Check sheet for the modelled part. Datum: model origin and axes. Units: mm. A direction names the side the tool comes from. Round coordinates to 2 decimals unless told otherwise and drop trailing zeros. Order: outer loops, then holes, each group sorted by start corner. A loop starts at its lowest first (then second) coordinate and runs counter-clockwise, first axis right, second up. Notation, with made-up numbers: (71.5, 37) -> (123.5, 37) arc R15 cw to (123.5, 48) -> close; hole circle Ø8 at (88, 51). An arc over 180 degrees is marked (long way). Use CSV: the item, a comma, the result in double quotes.
```python
from build123d import *

# Parameters (mm, degrees)
SKETCH2_R           = 14
BOSS_EXTRUDE1_DEPTH = 4
SKETCH1_W           = 8
SKETCH1_H           = 22.649954628
SKETCH1_W_2         = 6
SKETCH1_H_2         = 18.4
BOSS_EXTRUDE2_DEPTH = 18
SKETCH3_W           = 8
SKETCH3_H           = 22.649954628
BOSS_EXTRUDE3_DEPTH = 2
SKETCH4_W           = 6
SKETCH4_H           = 18.4
CUT_EXTRUDE1_DEPTH  = 29.142494559
SKETCH5_W           = 5
SKETCH5_H           = 18.4
CUT_EXTRUDE2_DEPTH  = 33.57299495
SKETCH11_W          = 8
SKETCH11_H          = 18.310644234
BOSS_EXTRUDE5_DEPTH = 5.5
BOSS_EXTRUDE4_DEPTH = 25.5
CUT_EXTRUDE4_START  = 5.5
SKETCH9_W           = 3.5
SKETCH9_H           = 7
CUT_EXTRUDE4_DEPTH  = 6
SKETCH7_R           = 0.75
CUT_EXTRUDE5_DEPTH  = 41.03022536
FILLET3_R           = 1
FILLET4_R           = 2
FILLET5_R           = 2
SKETCH14_W          = 1.5
SKETCH14_H          = 2
FILLET6_R           = 2


# Some blends are built 0.0001 mm under size
with BuildPart() as part:
    # Sketch2 → Boss-Extrude1 (new body)
    with BuildSketch(Plane.XY):
        Circle(SKETCH2_R)
    extrude(amount=BOSS_EXTRUDE1_DEPTH)

    # Sketch1 → Boss-Extrude2 (add)
    with BuildSketch(Plane.XY.offset(4)):
        Rectangle(SKETCH1_W, SKETCH1_H)
        Rectangle(SKETCH1_W_2, SKETCH1_H_2, mode=Mode.SUBTRACT)
    extrude(amount=BOSS_EXTRUDE2_DEPTH)

    # Sketch3 → Boss-Extrude3 (add)
    with BuildSketch(Plane.XY.offset(22)):
        Rectangle(SKETCH3_W, SKETCH3_H)
    extrude(amount=BOSS_EXTRUDE3_DEPTH)

    # Sketch4 → Cut-Extrude1 (cut, through all)
    with BuildSketch(Plane.XY.offset(4)):
        Rectangle(SKETCH4_W, SKETCH4_H)
    extrude(amount=-CUT_EXTRUDE1_DEPTH, mode=Mode.SUBTRACT)

    # Sketch5 → Cut-Extrude2 (cut, through all)
    with BuildSketch(Plane.ZY.offset(-3)):
        with Locations((19.5, 0)):
            Rectangle(SKETCH5_W, SKETCH5_H)
    extrude(amount=CUT_EXTRUDE2_DEPTH, mode=Mode.SUBTRACT)

    # Sketch11 → Boss-Extrude5 (add)
    with BuildSketch(Plane.XY.offset(24)):
        Rectangle(SKETCH11_W, SKETCH11_H)
    extrude(amount=BOSS_EXTRUDE5_DEPTH)

    # Sketch8 → Boss-Extrude4 (add)
    with BuildSketch(Plane.XY.offset(4)):
        with BuildLine():
            Line((4, 11.324977314), (4, -11.324977314))
            Line((4, -11.324977314), (8.23072833, -11.324977314))
            ThreePointArc((8.23072833, -11.324977314), (12.474578081, -6.354911619), (14, 0))
            ThreePointArc((14, 0), (12.474578081, 6.354911619), (8.23072833, 11.324977314))
            Line((8.23072833, 11.324977314), (4, 11.324977314))
        make_face()
    extrude(amount=BOSS_EXTRUDE4_DEPTH)

    # Sketch9 → Cut-Extrude4 (cut)
    with BuildSketch(Plane.XY.offset(24).offset(CUT_EXTRUDE4_START)):
        with Locations((5.75, 0)):
            Rectangle(SKETCH9_W, SKETCH9_H)
    extrude(amount=-CUT_EXTRUDE4_DEPTH, mode=Mode.SUBTRACT)

    # Sketch7 → Cut-Extrude5 (cut, through all)
    with BuildSketch(Plane(origin=(0, -9.155322117, 0), x_dir=(1, 0, 0), z_dir=(0, 1, 0))):
        with Locations((0, -26.75)):
            Circle(SKETCH7_R)
    extrude(amount=CUT_EXTRUDE5_DEPTH, mode=Mode.SUBTRACT)

    # Fillet3
    fillet3_edges = [part.edges().sort_by_distance(p)[0] for p in [
        (-4, -9.2, 19.5),
        (-4, 0, 17),
        (-4, 9.2, 19.5),
    ]]
    fillet(fillet3_edges, radius=FILLET3_R - 0.0001)  # a hair under: the kernel refuses the full size

    # Fillet4
    # the kernel refuses this fillet: 2 mm, written as the material it adds along each edge
    with BuildSketch(Plane(origin=(13.23072833, -11.324977314, 4), x_dir=(0, -1, 0), z_dir=(-1, 0, 0))) as fillet4_piece_1_section:
        with BuildLine():
            CenterArc((FILLET4_R, FILLET4_R), FILLET4_R, 180, 90)
            Line((0, FILLET4_R), (0, 0))
            Line((0, 0), (FILLET4_R, 0))
        make_face()
    fillet4_piece_1 = extrude(amount=17.23072833, mode=Mode.PRIVATE)
    fillet4_piece_1 = fillet4_piece_1 & Plane(origin=(0, 0, 4.46853923), x_dir=(1, 0, 0), z_dir=(0, 0, -1)) * Cylinder(14, 43, mode=Mode.PRIVATE)
    add(fillet4_piece_1)
    with BuildSketch(Plane(origin=(-4, 11.324977314, 4), x_dir=(0, 0, 1), z_dir=(0, -1, 0))) as fillet4_piece_2:
        with BuildLine():
            CenterArc((FILLET4_R, FILLET4_R), FILLET4_R, 180, 90)
            Line((0, FILLET4_R), (0, 0))
            Line((0, 0), (FILLET4_R, 0))
        make_face()
    extrude(amount=22.649954628)
    with BuildSketch(Plane(origin=(-4, 11.324977314, 4), x_dir=(0, 1, 0), z_dir=(1, 0, 0))) as fillet4_piece_3_section:
        with BuildLine():
            CenterArc((FILLET4_R, FILLET4_R), FILLET4_R, 180, 90)
            Line((0, FILLET4_R), (0, 0))
            Line((0, 0), (FILLET4_R, 0))
        make_face()
    fillet4_piece_3 = extrude(amount=17.23072833, mode=Mode.PRIVATE)
    fillet4_piece_3 = fillet4_piece_3 & Plane(origin=(0, 0, 4.468539385), x_dir=(1, 0, 0), z_dir=(0, 0, -1)) * Cylinder(14, 43, mode=Mode.PRIVATE)
    add(fillet4_piece_3)
    with BuildSketch(Plane(origin=(-4, 11.324977314, 4), x_dir=(0, 0, 1), z_dir=(0, -1, 0))) as fillet4_piece_4a_section:
        with BuildLine():
            CenterArc((FILLET4_R, FILLET4_R), FILLET4_R, 180, 90)
            Line((0, FILLET4_R), (0, 0))
            Line((0, 0), (FILLET4_R, 0))
        make_face()
    fillet4_piece_4a = extrude(amount=27.649954628, mode=Mode.PRIVATE)
    fillet4_piece_4a = split(fillet4_piece_4a, bisect_by=Plane(origin=(-4.418611248, -11.324977314, 4.472457753), z_dir=(0, -1, 0)), keep=Keep.TOP, mode=Mode.PRIVATE)
    fillet4_piece_4a = fillet4_piece_4a & Plane(origin=(0, 0, 4.472457753), x_dir=(1, 0, 0), z_dir=(0, 0, -1)) * Cylinder(14, 64, mode=Mode.PRIVATE)
    with BuildSketch(Plane(origin=(13.23072833, -11.324977314, 4), x_dir=(0, -1, 0), z_dir=(-1, 0, 0))) as fillet4_piece_4b_section:
        with BuildLine():
            CenterArc((FILLET4_R, FILLET4_R), FILLET4_R, 180, 90)
            Line((0, FILLET4_R), (0, 0))
            Line((0, 0), (FILLET4_R, 0))
        make_face()
    fillet4_piece_4b = extrude(amount=22.23072833, mode=Mode.PRIVATE)
    fillet4_piece_4b = split(fillet4_piece_4b, bisect_by=Plane(origin=(-4, -11.687205264, 4.504335867), z_dir=(-1, 0, 0)), keep=Keep.TOP, mode=Mode.PRIVATE)
    fillet4_piece_4b = fillet4_piece_4b & Plane(origin=(0, 0, 4.504335867), x_dir=(1, 0, 0), z_dir=(0, 0, -1)) * Cylinder(14, 53, mode=Mode.PRIVATE)
    fillet4_piece_4 = fillet4_piece_4a & fillet4_piece_4b
    add(fillet4_piece_4)
    with BuildSketch(Plane(origin=(-4, 16.324977314, 4), x_dir=(0, 0, 1), z_dir=(0, -1, 0))) as fillet4_piece_5a_section:
        with BuildLine():
            CenterArc((FILLET4_R, FILLET4_R), FILLET4_R, 180, 90)
            Line((0, FILLET4_R), (0, 0))
            Line((0, 0), (FILLET4_R, 0))
        make_face()
    fillet4_piece_5a = extrude(amount=27.649954628, mode=Mode.PRIVATE)
    fillet4_piece_5a = split(fillet4_piece_5a, bisect_by=Plane(origin=(-4.418615633, 11.324977314, 4.472459709), z_dir=(0, 1, 0)), keep=Keep.TOP, mode=Mode.PRIVATE)
    fillet4_piece_5a = fillet4_piece_5a & Plane(origin=(0, 0, 4.472459709), x_dir=(1, 0, 0), z_dir=(0, 0, -1)) * Cylinder(14, 64, mode=Mode.PRIVATE)
    with BuildSketch(Plane(origin=(-9, 11.324977314, 4), x_dir=(0, 1, 0), z_dir=(1, 0, 0))) as fillet4_piece_5b_section:
        with BuildLine():
            CenterArc((FILLET4_R, FILLET4_R), FILLET4_R, 180, 90)
            Line((0, FILLET4_R), (0, 0))
            Line((0, 0), (FILLET4_R, 0))
        make_face()
    fillet4_piece_5b = extrude(amount=22.23072833, mode=Mode.PRIVATE)
    fillet4_piece_5b = split(fillet4_piece_5b, bisect_by=Plane(origin=(-4, 11.687206224, 4.504336165), z_dir=(-1, 0, 0)), keep=Keep.TOP, mode=Mode.PRIVATE)
    fillet4_piece_5b = fillet4_piece_5b & Plane(origin=(0, 0, 4.504336165), x_dir=(1, 0, 0), z_dir=(0, 0, -1)) * Cylinder(14, 53, mode=Mode.PRIVATE)
    fillet4_piece_5 = fillet4_piece_5a & fillet4_piece_5b
    add(fillet4_piece_5)

    # Fillet5
    fillet5_edges = [part.edges().sort_by_distance(p)[0] for p in [
        (3, 0, 22),
    ]]
    fillet(fillet5_edges, radius=FILLET5_R)

    # Sketch14 → Cut-Revolve1 (revolve, cut)
    with BuildSketch(Plane(origin=(0, 0, 0), x_dir=(1, 0, 0), z_dir=(0, 1, 0))):
        Polygon((10.5, -2), (10.5, -29.5), (13, -29.5), (13, -3.6), (12, -2), align=None)
        with Locations((11.25, -1)):
            Rectangle(SKETCH14_W, SKETCH14_H)
    cut_revolve1 = revolve(axis=Axis((10.5, 0, 29.5), (0, 0, -1)), mode=Mode.SUBTRACT)

    # Mirror1: Cut-Revolve1 across plane
    add(cut_revolve1.mirror(Plane(origin=(0, 0, 0), x_dir=(0, 0, 1), z_dir=(1, 0, 0))), mode=Mode.SUBTRACT)

    # Fillet6
    # the kernel refuses this fillet: 2 mm, written as the material it adds along each edge
    with BuildSketch(Plane(origin=(4, -11.324977314, 24), x_dir=(-1, 0, 0), z_dir=(0, 1, 0)), Plane(origin=(4, 4.155322117, 24), x_dir=(-1, 0, 0), z_dir=(0, 1, 0))) as fillet6_piece_1:
        with BuildLine():
            CenterArc((FILLET6_R, FILLET6_R), FILLET6_R, 180, 90)
            Line((0, FILLET6_R), (0, 0))
            Line((0, 0), (FILLET6_R, 0))
        make_face()
    extrude(amount=7.169655197)
    # the kernel refuses this fillet: 2 mm, written as the material it takes off along each edge
    with BuildSketch(Plane(origin=(4, 16.324977314, 29.5), x_dir=(1, 0, 0), z_dir=(0, -1, 0)), Plane(origin=(4, -9.155322117, 29.5), x_dir=(1, 0, 0), z_dir=(0, -1, 0))) as fillet6_2_piece_1:
        with BuildLine():
            CenterArc((FILLET6_R, -FILLET6_R), FILLET6_R, 90, 90)
            Line((0, -FILLET6_R), (0, 0))
            Line((0, 0), (FILLET6_R, 0))
        make_face()
    extrude(amount=7.169655197, mode=Mode.SUBTRACT)
    with BuildSketch(Plane(origin=(7.5, 3.5, 29.5), x_dir=(0, 1, 0), z_dir=(-1, 0, 0)), Plane(origin=(4, -3.5, 29.5), x_dir=(0, -1, 0), z_dir=(1, 0, 0))) as fillet6_2_piece_2:
        with BuildLine():
            CenterArc((FILLET6_R, FILLET6_R), FILLET6_R, 180, 90)
            Line((0, FILLET6_R), (0, 0))
            Line((0, 0), (FILLET6_R, 0))
        make_face()
    extrude(amount=3.5, mode=Mode.SUBTRACT)
    with BuildSketch(Plane(origin=(7.5, -3.5, 29.5), x_dir=(1, 0, 0), z_dir=(0, 1, 0))) as fillet6_2_piece_3:
        with BuildLine():
            CenterArc((FILLET6_R, FILLET6_R), FILLET6_R, 180, 90)
            Line((0, FILLET6_R), (0, 0))
            Line((0, 0), (FILLET6_R, 0))
        make_face()
    extrude(amount=7, mode=Mode.SUBTRACT)
    with BuildSketch(Plane(origin=(-4, 14.155322117, 29.5), x_dir=(0, 0, -1), z_dir=(0, -1, 0))) as fillet6_2_piece_4:
        with BuildLine():
            CenterArc((FILLET6_R, FILLET6_R), FILLET6_R, 180, 90)
            Line((0, FILLET6_R), (0, 0))
            Line((0, 0), (FILLET6_R, 0))
        make_face()
    extrude(amount=28.310644234, mode=Mode.SUBTRACT)
    with BuildSketch(Plane(origin=(12.5, 3.5, 29.5), x_dir=(0, 1, 0), z_dir=(-1, 0, 0))) as fillet6_2_piece_5a_section:
        with BuildLine():
            CenterArc((FILLET6_R, FILLET6_R), FILLET6_R, 180, 90)
            Line((0, FILLET6_R), (0, 0))
            Line((0, 0), (FILLET6_R, 0))
        make_face()
    fillet6_2_piece_5a = extrude(amount=8.5, mode=Mode.PRIVATE)
    fillet6_2_piece_5a = split(fillet6_2_piece_5a, bisect_by=Plane(origin=(7.5, 3.952790229, 29.047209771), z_dir=(1, 0, 0)), keep=Keep.TOP, mode=Mode.PRIVATE)
    with BuildSketch(Plane(origin=(7.5, -3.5, 29.5), x_dir=(1, 0, 0), z_dir=(0, 1, 0))) as fillet6_2_piece_5b_section:
        with BuildLine():
            CenterArc((FILLET6_R, FILLET6_R), FILLET6_R, 180, 90)
            Line((0, FILLET6_R), (0, 0))
            Line((0, 0), (FILLET6_R, 0))
        make_face()
    fillet6_2_piece_5b = extrude(amount=12, mode=Mode.PRIVATE)
    fillet6_2_piece_5b = split(fillet6_2_piece_5b, bisect_by=Plane(origin=(7.952790229, 3.5, 29.047209771), z_dir=(0, 1, 0)), keep=Keep.TOP, mode=Mode.PRIVATE)
    fillet6_2_piece_5 = fillet6_2_piece_5a & fillet6_2_piece_5b
    add(fillet6_2_piece_5, mode=Mode.SUBTRACT)
    with BuildSketch(Plane(origin=(4, -3.5, 29.5), x_dir=(0, -1, 0), z_dir=(1, 0, 0))) as fillet6_2_piece_6a_section:
        with BuildLine():
            CenterArc((FILLET6_R, FILLET6_R), FILLET6_R, 180, 90)
            Line((0, FILLET6_R), (0, 0))
            Line((0, 0), (FILLET6_R, 0))
        make_face()
    fillet6_2_piece_6a = extrude(amount=8.5, mode=Mode.PRIVATE)
    fillet6_2_piece_6a = split(fillet6_2_piece_6a, bisect_by=Plane(origin=(7.5, -3.952790229, 29.047209771), z_dir=(1, 0, 0)), keep=Keep.TOP, mode=Mode.PRIVATE)
    with BuildSketch(Plane(origin=(7.5, -8.5, 29.5), x_dir=(1, 0, 0), z_dir=(0, 1, 0))) as fillet6_2_piece_6b_section:
        with BuildLine():
            CenterArc((FILLET6_R, FILLET6_R), FILLET6_R, 180, 90)
            Line((0, FILLET6_R), (0, 0))
            Line((0, 0), (FILLET6_R, 0))
        make_face()
    fillet6_2_piece_6b = extrude(amount=12, mode=Mode.PRIVATE)
    fillet6_2_piece_6b = split(fillet6_2_piece_6b, bisect_by=Plane(origin=(7.952790229, -3.5, 29.047209771), z_dir=(0, -1, 0)), keep=Keep.TOP, mode=Mode.PRIVATE)
    fillet6_2_piece_6 = fillet6_2_piece_6a & fillet6_2_piece_6b
    add(fillet6_2_piece_6, mode=Mode.SUBTRACT)


solid = part.part
```
Q1. Sectioned sample at B-B, the plane x = 0. Enter the section's corners in (y, z), then the cut area to 3 significant figures.
Result sheet:
outline,"(-14, 0) -> (-9.2, 0) -> (-9.2, 22) -> (9.2, 22) -> (9.2, 0) -> (14, 0) -> (14, 4) -> (13.32, 4) arc R2 cw to (11.32, 6) -> (11.32, 24) -> (9.16, 24) -> (9.16, 26) -> (-9.16, 26) -> (-9.16, 24) -> (-11.32, 24) -> (-11.32, 6) arc R2 cw to (-13.32, 4) -> (-14, 4) -> close; (-9.16, 27.5) -> (9.16, 27.5) -> (9.16, 29.5) -> (-9.16, 29.5) -> close"
area,"235 mm^2"
Q2. Mould release check, pull along Z, two halves, no side actions. Record for faces 1 (the face through (4.6, 10.26, 28.93)), 2 (the face through (6, -3.5, 26)), 3 (the face through (-3.715, -9.501, 18.958)): pulls with the +Z half, pulls with the -Z half, needs draft (parallel to the pull), parting line crosses it, or undercut.
Result sheet:
face 1,"pulls with the +Z half"
face 2,"needs draft"
face 3,"undercut"
Q3. Access from +Z, -Z, +X, -X, +Y, -Y to the whole of each face (thin tool, end or side, straight path). Record for faces 4 (the face through (6, 0, 23.5)), 5 (the face through (-1, -10, 24)), 6 (the face through (0, -9.2, 11)), 7 (the face through (2, -11.325, 15)).
Result sheet:
face 4,"+Z"
face 5,"+Z, -X, -Y"
face 6,"-Z"
face 7,"+Z, +X, -X, -Y"
Q4. Sectioned sample at A-A, the plane y = 6. State how many separate pieces and enclosed holes the cut face has, then the cut area to 3 significant figures.
Result sheet:
separate pieces,"2"
enclosed holes,"1"
area,"388 mm^2"
Q5. Scan lines: L1, parallel to X at y = 0, z = 3.8; L2, parallel to Y at x = 2.25, z = 14.25; L3, parallel to Z at x = 0, y = 1.5. Record each from-to range of solid material in increasing order.
Result sheet:
L1,"x = -14 to -13, -8 to -3, 3 to 8, 13 to 14"
L2,"y = -11.32 to -9.2, 9.2 to 11.32"
L3,"z = 22 to 26, 27.5 to 29.5"
Q6. Sectioned sample at C-C, the plane z = 6.5. Enter the section's corners in (x, y), then the cut area to 3 significant figures.
Result sheet:
outline,"(-4, -11.32) -> (8.23, -11.32) arc R14 ccw to (8.23, 11.32) -> (-4, 11.32) -> close; hole (-3, -9.2) -> (3, -9.2) -> (3, 9.2) -> (-3, 9.2) -> close; hole circle Ø5 at (10.5, 0)"
area,"238 mm^2"
Q7. Go/stop test with flat-tipped pins: pin 1 (6 mm diameter, centred on x = 1, z = 15.5, fed in from +Y) (3 decimals); pin 2 (6 mm diameter, centred on x = -1, z = 28, fed in from +Y); pin 3 (0.5 mm diameter, centred on x = -1.5, y = -13.5, fed in from +Z); pin 4 (5 mm diameter, centred on x = -2.5, y = -5.5, fed in from -Z). Record where each tip stops, or that it passes through.
Result sheet:
pin 1,"stops at y = 11.325"
pin 2,"stops at y = 9.16"
pin 3,"stops at z = 4"
pin 4,"stops at z = 0"
